The model under review builds one solid part; all positions refer to its coordinate system, in mm. A direction names the side the tool comes from. Coordinates: 2 decimals unless noted, no trailing zeros. Order: outer loops, then holes, each group sorted by start corner. A loop starts at its lowest first (then second) coordinate and runs counter-clockwise, first axis right, second up. Notation, with made-up numbers: M 72.25,39 L 122.25,39 A9 cw 122.25,46 Z; hole C 13.25,82 d9. An arc over 180 degrees is marked long. Answer in a Markdown table with one row per item.
from build123d import *

# Parameters (mm, degrees)
BOSS_EXTRUDE1_DEPTH = 62
FILLET1_R           = 6
FILLET2_R           = 6
CAVITY1_START       = -1.5
CAVITY1_OUTLINE_W   = 50
CAVITY1_OUTLINE_H   = 15
CAVITY1_DEPTH       = 3
SKETCH2_W           = 132.712401986
SKETCH2_H           = 25.545070458
CUT_EXTRUDE1_DEPTH  = 10


# Read off the part's stored shape, not the designer's step: Cavity1
with BuildPart() as part:
    # Sketch1 → Boss-Extrude1 (new body)
    with BuildSketch(Plane(origin=(0, 0, 0), x_dir=(0, 0, -1), z_dir=(1, 0, 0))):
        with BuildLine():
            Line((-1.5, -7.5), (1.5, -7.5))
            ThreePointArc((1.5, -7.5), (5.742640687, -5.742640687), (7.5, -1.5))
            Line((7.5, -1.5), (7.5, 1.5))
            ThreePointArc((7.5, 1.5), (5.742640687, 5.742640687), (1.5, 7.5))
            Line((1.5, 7.5), (-1.5, 7.5))
            ThreePointArc((-1.5, 7.5), (-5.742640687, 5.742640687), (-7.5, 1.5))
            Line((-7.5, 1.5), (-7.5, -1.5))
            ThreePointArc((-7.5, -1.5), (-5.742640687, -5.742640687), (-1.5, -7.5))
        make_face()
    extrude(amount=BOSS_EXTRUDE1_DEPTH)

    # Fillet1
    fillet1_edges = [part.edges().sort_by_distance(p)[0] for p in [
        (0, 7.5, 0),
        (0, 5.742640687, -5.742640687),
        (0, 0, -7.5),
        (0, -5.742640687, -5.742640687),
        (0, -7.5, 0),
        (0, -5.742640687, 5.742640687),
        (0, 0, 7.5),
        (0, 5.742640687, 5.742640687),
    ]]
    fillet(fillet1_edges, radius=FILLET1_R)

    # Fillet2
    fillet2_edges = [part.edges().sort_by_distance(p)[0] for p in [
        (62, 5.742640687, -5.742640687),
        (62, 7.5, 0),
        (62, 5.742640687, 5.742640687),
        (62, 0, 7.5),
        (62, -5.742640687, 5.742640687),
        (62, -7.5, 0),
        (62, -5.742640687, -5.742640687),
        (62, 0, -7.5),
    ]]
    fillet(fillet2_edges, radius=FILLET2_R)

    # Cavity1 outline → Cavity1 (cut)
    with BuildSketch(Plane(origin=(0, 0, 0), x_dir=(1, 0, 0), z_dir=(0, 1, 0)).offset(CAVITY1_START)):
        with Locations((31, 0)):
            Rectangle(CAVITY1_OUTLINE_W, CAVITY1_OUTLINE_H)
    extrude(amount=CAVITY1_DEPTH, mode=Mode.SUBTRACT)

    # Sketch2 → Cut-Extrude1 (cut)
    with BuildSketch(Plane(origin=(0, 0, 0), x_dir=(1, 0, 0), z_dir=(0, 1, 0))):
        Rectangle(SKETCH2_W, SKETCH2_H)
    extrude(amount=CUT_EXTRUDE1_DEPTH, mode=Mode.SUBTRACT)


solid = part.part
(1) Take a section at A-A (z = -0.75). Write out the cut boundary in (x, y), then the cut area to 3 significant figures.
Report:
| item | result |
|---|---|
| outline | M 0,-1.5 A6 ccw 6,-7.5 L 56,-7.5 A6 ccw 62,-1.5 L 62,0 L 56,0 L 56,-1.5 L 6,-1.5 L 6,0 L 0,0 Z |
| area | 375 mm^2 |
(2) To check wall thickness, follow line 1 (Y direction, x = 51.5, z = -0.5); line 2 (Z direction, x = 38.5, y = -1.75); line 3 (X direction, y = -0.75, z = -5.25). State the ranges of each line that lie inside material, in increasing order. Write a range as [from, to].
Report:
| item | result |
|---|---|
| line 1 | [-7.5, -1.5] |
| line 2 | [-7.49, 7.49] |
| line 3 | [1.32, 6], [56, 60.68] |
(3) Machinability: for faces 5 (the flat face through (58, 0, 0)), 6 (the flat face through (31, -1.5, 0)), which of the approach directions +Z, -Z, +X, -X, +Y, -Y give a long, thin tool a straight path to every point of the face, cutting with its end or side? Answer none if there is none.
Report:
| item | result |
|---|---|
| face 5 | +Z, -Z, +X, -X, +Y |
| face 6 | +Z, -Z, +Y |
(4) Insertion check: P1, Ø3, axis at x = 21, y = -3.5, coming from the -Z side; P2, Ø4, axis at x = 8, z = -4, coming from the -Y side; P3, Ø1, axis at y = -3, z = 0.5, coming from the +X side. Each pin has a flat end and moves straight along its axis. Give the tip position at first contact, or say it passes through.
Report:
| item | result |
|---|---|
| P1 | z = -7.48 |
| P2 | y = -7.48 |
| P3 | x = 61.92 |
(5) The part is to be moulded in two halves that separate along X. For faces 1 (the flat face through (56, -1, 0)), 2 (the cylindrical face through (30.65, -5.696, 5.789)), 3 (the cylindrical face through (60.289, -0.76, 5.696)), 4 (the flat face through (6, -1, 0)), say which applies: +X half, -X half, draft (parallel to the pull), parting line (faces both ways), or undercut.
Report:
| item | result |
|---|---|
| face 1 | undercut |
| face 2 | draft |
| face 3 | +X half |
| face 4 | undercut |
(6) Take a section at B-B (y = -2.5). Write out the cut boundary in (x, z).
Report:
| item | result |
|---|---|
| outline | M 0.08,-1.5 A5.92 ccw 6,-7.42 L 56,-7.42 A5.92 ccw 61.92,-1.5 L 61.92,1.5 A5.92 ccw 56,7.42 L 6,7.42 A5.92 ccw 0.08,1.5 Z |
(7) Take a section at D-D (y = -5). Write out the cut boundary in (x, z), then the cut area to 3 significant figures.
Report:
| item | result |
|---|---|
| outline | M 1.13,-1.5 A4.87 ccw 6,-6.37 L 56,-6.37 A4.87 ccw 60.87,-1.5 L 60.87,1.5 A4.87 ccw 56,6.37 L 6,6.37 A4.87 ccw 1.13,1.5 Z |
| area | 741 mm^2 |
(8) Take a section at C-C (x = 8). Write out the cut boundary in (y, z), then the cut area to 3 significant figures.
Report:
| item | result |
|---|---|
| outline | M -7.5,-1.5 A6 ccw -1.5,-7.5 L -1.5,7.5 A6 ccw -7.5,1.5 Z |
| area | 74.5 mm^2 |
